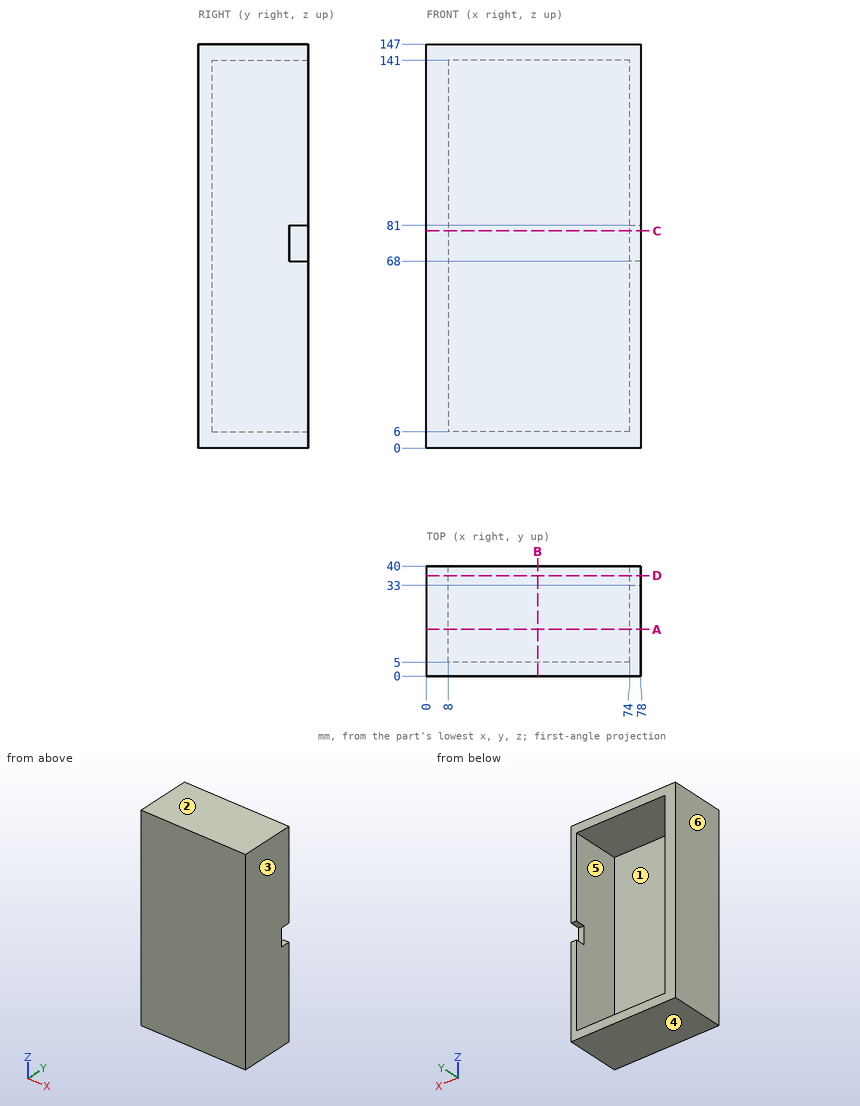
Check sheet for the drawn part. Datum: minimum x, y, z corner. Units: mm. A direction names the side the tool comes from. Round coordinates to 2 decimals unless told otherwise and drop trailing zeros. Order: outer loops, then holes, each group sorted by start corner. A loop starts at its lowest first (then second) coordinate and runs counter-clockwise, first axis right, second up. Notation, with made-up numbers: (-4, 89.5) -> (22, 89.5) arc R17 ccw to (22, 109.5) -> close; hole circle Ø10 at (83.5, 20). An arc over 180 degrees is marked (long way). Use CSV: the item, a comma, the result in double quotes.
(1) Material ranges on line 1 along Z through (x, y) = (63, 37.5); line 2 along X through (y, z) = (10.5, 32); line 3 along Y through (x, z) = (12, 137.5), recorded low to high. Write a range as from..to.
Worked out:
line 1,"0..6, 141..147"
line 2,"0..8, 74..78"
line 3,"0..5"
(2) Cross-section at A-A (y = 17). Record the boundary of the cut face in (x, z).
Worked out:
outline,"(0, 0) -> (78, 0) -> (78, 147) -> (0, 147) -> close; hole (8, 6) -> (74, 6) -> (74, 141) -> (8, 141) -> close"
(3) Cross-section at D-D (y = 36.5). Record the boundary of the cut face in (x, z).
Worked out:
outline,"(0, 0) -> (78, 0) -> (78, 68) -> (74, 68) -> (74, 6) -> (8, 6) -> (8, 141) -> (74, 141) -> (74, 81) -> (78, 81) -> (78, 147) -> (0, 147) -> close"
(4) Cross-section at B-B (x = 40.5). Record the boundary of the cut face in (y, z), and give its area (4 significant figures).
Worked out:
outline,"(0, 0) -> (40, 0) -> (40, 6) -> (5, 6) -> (5, 141) -> (40, 141) -> (40, 147) -> (0, 147) -> close"
area,"1,155 mm²"
(5) Cross-section at C-C (z = 79). Record the boundary of the cut face in (x, y).
Worked out:
outline,"(0, 0) -> (78, 0) -> (78, 33) -> (74, 33) -> (74, 5) -> (8, 5) -> (8, 40) -> (0, 40) -> close"
(6) Draft check along X on the marked faces 3, 4, 5 and 6. Enter one of: pulls with the +X half, pulls with the -X half, needs draft (parallel to the pull), parting line crosses it, or undercut.
Worked out:
face 3,"pulls with the +X half"
face 4,"needs draft"
face 5,"undercut"
face 6,"pulls with the -X half"
(7) Depth check by flat-ended pin: pin 1 (4.5 mm diameter, centred on x = 75, z = 71.5, fed in from +Y). Enter the tip coordinate at first touch or a pass-through.
Worked out:
pin 1,"y = 33"
(8) Tool access check on the marked faces 1 and 2. Record the directions out of +Z, -Z, +X, -X, +Y, -Y that give a thin tool (end or side, any length) a straight path to the whole face; none if there is none.
Worked out:
face 1,"+Y"
face 2,"+Z, +X, -X, +Y, -Y"
